from build123d import *

# Parameters (mm, degrees)
BOSS_EXTRUDE1_DEPTH = 33.02


with BuildPart() as part:
    # Sketch1 → Boss-Extrude1 (new body)
    with BuildSketch(Plane.XY):
        with BuildLine():
            ThreePointArc((-5.305232227, 13.252552057), (-7.1375, 12.362512639), (-8.824430633, 11.22074191))
            ThreePointArc((-8.824430633, 11.22074191), (-9.981957879, 10.782799599), (-11.181776449, 11.08627644))
            ThreePointArc((-11.181776449, 11.08627644), (-12.622148396, 11.355295802), (-13.870578082, 10.588180375))
            ThreePointArc((-13.870578082, 10.588180375), (-15.112143296, 8.725), (-16.104922226, 6.718182797))
            ThreePointArc((-16.104922226, 6.718182797), (-16.145048829, 5.25345326), (-15.191885255, 4.140564245))
            ThreePointArc((-15.191885255, 4.140564245), (-14.329157316, 3.253229304), (-14.12966286, 2.031810147))
            ThreePointArc((-14.12966286, 2.031810147), (-14.238619356, 1.01850078), (-14.275, 0))
            ThreePointArc((-14.275, 0), (-14.238619356, -1.01850078), (-14.12966286, -2.031810147))
            ThreePointArc((-14.12966286, -2.031810147), (-14.329157316, -3.253229304), (-15.191885255, -4.140564245))
            ThreePointArc((-15.191885255, -4.140564245), (-16.145048829, -5.25345326), (-16.104922226, -6.718182797))
            ThreePointArc((-16.104922226, -6.718182797), (-15.112143296, -8.725), (-13.870578082, -10.588180375))
            ThreePointArc((-13.870578082, -10.588180375), (-12.622148396, -11.355295802), (-11.181776449, -11.08627644))
            ThreePointArc((-11.181776449, -11.08627644), (-9.981957879, -10.782799599), (-8.824430633, -11.22074191))
            ThreePointArc((-8.824430633, -11.22074191), (-7.1375, -12.362512639), (-5.305232227, -13.252552057))
            ThreePointArc((-5.305232227, -13.252552057), (-4.347199437, -14.036028902), (-4.010108806, -15.226840684))
            ThreePointArc((-4.010108806, -15.226840684), (-3.522900434, -16.608749062), (-2.234344144, -17.306363172))
            ThreePointArc((-2.234344144, -17.306363172), (0, -17.45), (2.234344144, -17.306363172))
            ThreePointArc((2.234344144, -17.306363172), (3.503647323, -16.630968906), (4.010957256, -15.285634521))
            ThreePointArc((4.010957256, -15.285634521), (4.010745132, -15.256234542), (4.010108806, -15.226840684))
            ThreePointArc((4.010108806, -15.226840684), (4.009464671, -15.197086165), (4.009249945, -15.167325448))
            ThreePointArc((4.009249945, -15.167325448), (4.363702952, -14.011262386), (5.305232227, -13.252552057))
            ThreePointArc((5.305232227, -13.252552057), (7.1375, -12.362512639), (8.824430633, -11.22074191))
            ThreePointArc((8.824430633, -11.22074191), (9.981957879, -10.782799599), (11.181776449, -11.08627644))
            ThreePointArc((11.181776449, -11.08627644), (12.622148396, -11.355295802), (13.870578082, -10.588180375))
            ThreePointArc((13.870578082, -10.588180375), (15.112143296, -8.725), (16.104922226, -6.718182797))
            ThreePointArc((16.104922226, -6.718182797), (16.2223271, -6.333751864), (16.261976436, -5.933753144))
            ThreePointArc((16.261976436, -5.933753144), (15.974119502, -4.889648077), (15.191885255, -4.140564245))
            ThreePointArc((15.191885255, -4.140564245), (14.400052997, -3.382289157), (14.10866406, -2.325372926))
            ThreePointArc((14.10866406, -2.325372926), (14.113920458, -2.1782165), (14.12966286, -2.031810147))
            ThreePointArc((14.12966286, -2.031810147), (14.275, 0), (14.12966286, 2.031810147))
            ThreePointArc((14.12966286, 2.031810147), (14.113920458, 2.1782165), (14.10866406, 2.325372926))
            ThreePointArc((14.10866406, 2.325372926), (14.400052997, 3.382289157), (15.191885255, 4.140564245))
            ThreePointArc((15.191885255, 4.140564245), (15.974119502, 4.889648077), (16.261976436, 5.933753144))
            ThreePointArc((16.261976436, 5.933753144), (16.2223271, 6.333751864), (16.104922226, 6.718182797))
            ThreePointArc((16.104922226, 6.718182797), (15.112143296, 8.725), (13.870578082, 10.588180375))
            ThreePointArc((13.870578082, 10.588180375), (12.622148396, 11.355295802), (11.181776449, 11.08627644))
            ThreePointArc((11.181776449, 11.08627644), (9.981957879, 10.782799599), (8.824430633, 11.22074191))
            ThreePointArc((8.824430633, 11.22074191), (7.1375, 12.362512639), (5.305232227, 13.252552057))
            ThreePointArc((5.305232227, 13.252552057), (4.363702952, 14.011262386), (4.009249945, 15.167325448))
            ThreePointArc((4.009249945, 15.167325448), (4.009464671, 15.197086165), (4.010108806, 15.226840684))
            ThreePointArc((4.010108806, 15.226840684), (4.010745132, 15.256234542), (4.010957256, 15.285634521))
            ThreePointArc((4.010957256, 15.285634521), (3.503647323, 16.630968906), (2.234344144, 17.306363172))
            ThreePointArc((2.234344144, 17.306363172), (0, 17.45), (-2.234344144, 17.306363172))
            ThreePointArc((-2.234344144, 17.306363172), (-3.522900434, 16.608749062), (-4.010108806, 15.226840684))
            ThreePointArc((-4.010108806, 15.226840684), (-4.347199437, 14.036028902), (-5.305232227, 13.252552057))
        make_face()
        with BuildLine():
            ThreePointArc((-4.715245806, 11.778756863), (-6.34375, 10.987697311), (-7.843079766, 9.972901084))
            ThreePointArc((-7.843079766, 9.972901084), (-9.891552176, 9.197875923), (-12.014867411, 9.734937956))
            ThreePointArc((-12.014867411, 9.734937956), (-12.332986369, 9.794353275), (-12.608713171, 9.624929009))
            ThreePointArc((-12.608713171, 9.624929009), (-13.737327968, 7.93125), (-14.639789617, 6.107001411))
            ThreePointArc((-14.639789617, 6.107001411), (-14.648651934, 5.783502863), (-14.438137279, 5.537711424))
            ThreePointArc((-14.438137279, 5.537711424), (-12.911370298, 3.967397506), (-12.558325571, 1.805855779))
            ThreePointArc((-12.558325571, 1.805855779), (-12.655165189, 0.905234932), (-12.6875, 0))
            ThreePointArc((-12.6875, 0), (-12.655165189, -0.905234932), (-12.558325571, -1.805855779))
            ThreePointArc((-12.558325571, -1.805855779), (-12.911370298, -3.967397506), (-14.438137279, -5.537711424))
            ThreePointArc((-14.438137279, -5.537711424), (-14.648651934, -5.783502863), (-14.639789617, -6.107001411))
            ThreePointArc((-14.639789617, -6.107001411), (-13.737327968, -7.93125), (-12.608713171, -9.624929009))
            ThreePointArc((-12.608713171, -9.624929009), (-12.332986369, -9.794353275), (-12.014867411, -9.734937956))
            ThreePointArc((-12.014867411, -9.734937956), (-9.891552176, -9.197875923), (-7.843079766, -9.972901084))
            ThreePointArc((-7.843079766, -9.972901084), (-6.34375, -10.987697311), (-4.715245806, -11.778756863))
            ThreePointArc((-4.715245806, -11.778756863), (-3.019818122, -13.165273429), (-2.423269868, -15.272649379))
            ThreePointArc((-2.423269868, -15.272649379), (-2.315665565, -15.577856137), (-2.031076446, -15.731930419))
            ThreePointArc((-2.031076446, -15.731930419), (0, -15.8625), (2.031076446, -15.731930419))
            ThreePointArc((2.031076446, -15.731930419), (2.311413344, -15.582763588), (2.423457256, -15.285634521))
            ThreePointArc((2.423457256, -15.285634521), (2.423410406, -15.279141274), (2.423269868, -15.272649379))
            ThreePointArc((2.423269868, -15.272649379), (2.422129945, -15.219992897), (2.421749945, -15.167325448))
            ThreePointArc((2.421749945, -15.167325448), (3.049024342, -13.1214442), (4.715245806, -11.778756863))
            ThreePointArc((4.715245806, -11.778756863), (6.34375, -10.987697311), (7.843079766, -9.972901084))
            ThreePointArc((7.843079766, -9.972901084), (9.891552176, -9.197875923), (12.014867411, -9.734937956))
            ThreePointArc((12.014867411, -9.734937956), (12.332986369, -9.794353275), (12.608713171, -9.624929009))
            ThreePointArc((12.608713171, -9.624929009), (13.737327968, -7.93125), (14.639789617, -6.107001411))
            ThreePointArc((14.639789617, -6.107001411), (14.665719527, -6.022096419), (14.674476436, -5.933753144))
            ThreePointArc((14.674476436, -5.933753144), (14.610900672, -5.703153252), (14.438137279, -5.537711424))
            ThreePointArc((14.438137279, -5.537711424), (13.036834166, -4.195794332), (12.52116406, -2.325372926))
            ThreePointArc((12.52116406, -2.325372926), (12.530466291, -2.064950652), (12.558325571, -1.805855779))
            ThreePointArc((12.558325571, -1.805855779), (12.6875, 0), (12.558325571, 1.805855779))
            ThreePointArc((12.558325571, 1.805855779), (12.530466291, 2.064950652), (12.52116406, 2.325372926))
            ThreePointArc((12.52116406, 2.325372926), (13.036834166, 4.195794332), (14.438137279, 5.537711424))
            ThreePointArc((14.438137279, 5.537711424), (14.610900672, 5.703153252), (14.674476436, 5.933753144))
            ThreePointArc((14.674476436, 5.933753144), (14.665719527, 6.022096419), (14.639789617, 6.107001411))
            ThreePointArc((14.639789617, 6.107001411), (13.737327968, 7.93125), (12.608713171, 9.624929009))
            ThreePointArc((12.608713171, 9.624929009), (12.332986369, 9.794353275), (12.014867411, 9.734937956))
            ThreePointArc((12.014867411, 9.734937956), (9.891552176, 9.197875923), (7.843079766, 9.972901084))
            ThreePointArc((7.843079766, 9.972901084), (6.34375, 10.987697311), (4.715245806, 11.778756863))
            ThreePointArc((4.715245806, 11.778756863), (3.049024342, 13.1214442), (2.421749945, 15.167325448))
            ThreePointArc((2.421749945, 15.167325448), (2.422129945, 15.219992897), (2.423269868, 15.272649379))
            ThreePointArc((2.423269868, 15.272649379), (2.423410406, 15.279141274), (2.423457256, 15.285634521))
            ThreePointArc((2.423457256, 15.285634521), (2.311413344, 15.582763588), (2.031076446, 15.731930419))
            ThreePointArc((2.031076446, 15.731930419), (0, 15.8625), (-2.031076446, 15.731930419))
            ThreePointArc((-2.031076446, 15.731930419), (-2.315665565, 15.577856137), (-2.423269868, 15.272649379))
            ThreePointArc((-2.423269868, 15.272649379), (-3.019818122, 13.165273429), (-4.715245806, 11.778756863))
        make_face(mode=Mode.SUBTRACT)
    extrude(amount=BOSS_EXTRUDE1_DEPTH)


solid = part.part
Build history of the part. All positions in model axes, mm. A direction names the side the tool comes from. Coordinates: 2 decimals unless noted, no trailing zeros. Order: outer loops, then holes, each group sorted by start corner. A loop starts at its lowest first (then second) coordinate and runs counter-clockwise, first axis right, second up. Notation, with made-up numbers: M 89.5,-7 L 107.5,-7 A14 ccw 107.5,4 Z; hole C 13.25,-2 d11. An arc over 180 degrees is marked long. One line per question, with ' | ' between items. Start each with the question number.
Q1. 3-axis set-ups, long thin cutter, end or side, ignore diameter. For faces 4 (the face through (13.72, -7.96, 16.28)), 5 (the face through (-16.138, -5.234, 16.279)): which of +Z, -Z, +X, -X, +Y, -Y reach the whole face in a straight line?
Q2. Probe L1, parallel to X at y = 11, z = 27; L2, parallel to Y at x = -14, z = 14; L3, parallel to Y at x = 10, z = 29.5. List the from-to ranges inside material, lowest first. Write a range as from..to.
Q3. Flat gauge pins, fed straight in: pin 1 Ø6 at (y, z) = (-0.5, 21.5) entering from +X; pin 2 Ø1 at (y, z) = (-3.5, 12) entering from -X; pin 3 Ø5 at (y, z) = (-12, 21.5) entering from -X. Where does each tip first touch, or does it go through?
Q4. Saw through at B-B (y = -3). List the corners of the cut face in (x, z), then the cut area to 3 significant figures.
Q5. Two-plate mould, pull along X, no slides. Class faces 1 (the face through (0.03, 17.45, 16.28)), 2 (the face through (-6, -12, 0)), 3 (the face through (-6.366, -10.975, 16.279)): +X half, -X half, draft (parallel to the pull), parting line (faces both ways), or undercut.
Q6. Saw through at A-A (x = -3.5). List the corners of the cut face in (y, z).
Check values:
1) face 4: +Z, -Z | face 5: +Z, -Z, -X
2) L1: x = -13.45..-11.03, -9.17..-6.32, 6.32..9.17, 11.03..13.45 | L2: y = -10.42..-7.46, -5.26..5.26, 7.46..10.42 | L3: y = -10.78..-9.19, 9.19..10.78
3) pin 1: stops at x = 14.48 | pin 2: stops at x = -14.97 | pin 3: stops at x = -14.64
4) outline: M -14.22,0 L -12.58,0 L -12.58,33.02 L -14.22,33.02 Z; M 12.58,0 L 14.22,0 L 14.22,33.02 L 12.58,33.02 Z | area: 108 mm2
5) face 1: parting line | face 2: draft | face 3: undercut
6) outline: M -16.64,0 L -12.58,0 L -12.58,33.02 L -16.64,33.02 Z; M 12.58,0 L 16.64,0 L 16.64,33.02 L 12.58,33.02 Z
